Geometry check sheet. Reference: drawing and pictorial views, mm from the part's lowest x, y, z. A direction names the side the tool comes from. Coordinates: 2 decimals unless noted, no trailing zeros. Write each loop counter-clockwise with the first axis right and the second up, starting at its lowest first coordinate (ties: lowest second). Pieces come first, ordered by that corner, then holes. Notation, with made-up numbers: (-10, 71.5) -> (-2, 71.5) arc R19 cw to (-2, 100.5) -> close; hole circle Ø3 at (11.5, 17). An arc over 180 degrees is marked (long way). Answer in a Markdown table with one row per item.
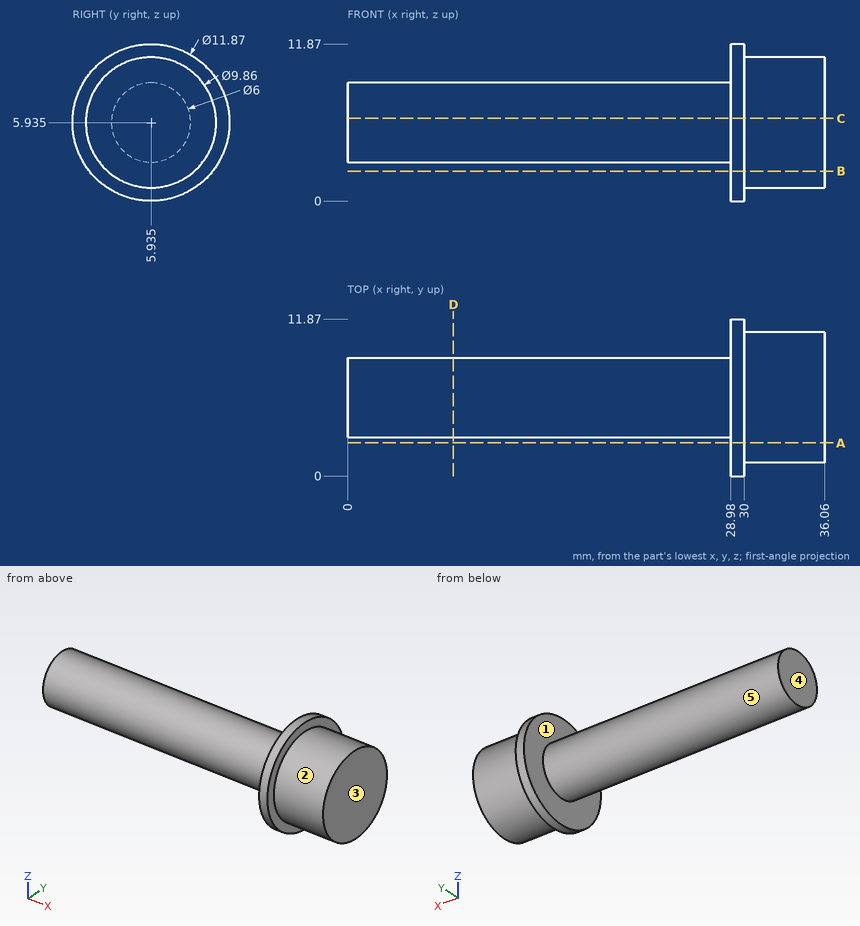
1. Section check D-D, the plane x = 8. Record the boundary of the cut face in (y, z) (3 decimals).
Geometry says:
| item | result |
|---|---|
| outline | circle Ø6 at (5.935, 5.935) |
2. Section check B-B, the plane z = 2.25. Record the boundary of the cut face in (x, y).
Geometry says:
| item | result |
|---|---|
| outline | (28.98, 1.28) -> (30, 1.28) -> (30, 2.66) -> (36.06, 2.66) -> (36.06, 9.21) -> (30, 9.21) -> (30, 10.59) -> (28.98, 10.59) -> close |
3. Depth check by flat-ended pin: P1, Ø6, axis at y = 9.5, z = 9.5, coming from the +X side; P2, Ø6, axis at x = 23, z = 3, coming from the -Y side (3 decimals); P3, Ø4, axis at x = 4.5, y = 6.5, coming from the +Z side (3 decimals); P4, Ø2, axis at x = 22, z = 5, coming from the +Y side (3 decimals). Enter the tip coordinate at first touch or a pass-through.
Geometry says:
| item | result |
|---|---|
| P1 | x = 36.06 |
| P2 | y = 2.935 |
| P3 | z = 8.935 |
| P4 | y = 8.935 |
4. Tool access check on the marked faces 1 and 2. Record the directions out of +Z, -Z, +X, -X, +Y, -Y that give a thin tool (end or side, any length) a straight path to the whole face; none if there is none.
Geometry says:
| item | result |
|---|---|
| face 1 | -X |
| face 2 | +X |
5. Thickness scan on line 1 (X direction, y = 4.75, z = 2); line 2 (X direction, y = 9.75, z = 2.5); line 3 (Y direction, x = 32, z = 4.25). Record the ranges inside material, lowest first. Write a range as from..to.
Geometry says:
| item | result |
|---|---|
| line 1 | 28.98..36.06 |
| line 2 | 28.98..30 |
| line 3 | 1.3..10.57 |
6. Mould release check, pull along X, two halves, no side actions. Record for the marked faces 3, 4 and 5: released by +X, released by -X, zero draft, split by the parting line, or undercut.
Geometry says:
| item | result |
|---|---|
| face 3 | released by +X |
| face 4 | released by -X |
| face 5 | zero draft |
7. Section check C-C, the plane z = 6.25. Record the boundary of the cut face in (x, y), plus the area to 3 significant figures.
Geometry says:
| item | result |
|---|---|
| outline | (0, 2.95) -> (28.98, 2.95) -> (28.98, 0.01) -> (30, 0.01) -> (30, 1.02) -> (36.06, 1.02) -> (36.06, 10.85) -> (30, 10.85) -> (30, 11.86) -> (28.98, 11.86) -> (28.98, 8.92) -> (0, 8.92) -> close |
| area | 245 mm^2 |
8. Section check A-A, the plane y = 2.5. Record the boundary of the cut face in (x, z), plus the area to 3 significant figures.
Geometry says:
| item | result |
|---|---|
| outline | (28.98, 1.1) -> (30, 1.1) -> (30, 2.4) -> (36.06, 2.4) -> (36.06, 9.47) -> (30, 9.47) -> (30, 10.77) -> (28.98, 10.77) -> close |
| area | 52.7 mm^2 |
